Input: dimensioned drawing with shaded views. Units: mm. Origin: part minimum x, y, z. A direction names the side the tool comes from. Round coordinates to 2 decimals unless told otherwise and drop trailing zeros. Loops run counter-clockwise (first coordinate to the right, second up) from the corner with the lowest first, then second, coordinate; pieces in that order, holes last. Notation, with made-up numbers: (88, -23.75) - (146, -23.75) arc R23 cw to (146, 5.25) - close; hole circle Ø8 at (62.25, 53). An arc over 180 degrees is marked (long way). One line per question, with ' | ' between items. Start each with the question number.
Item 1: Section B-B, the plane x = 72.5. Return loops of the section in (y, z) (3 decimals), plus the area to 3 significant figures.
Item 2: Material intervals for line 1 along X through (y, z) = (7.5, 20); line 2 along X through (y, z) = (19, 20); line 3 along Z through (x, y) = (78.5, 20.5), sorted ascending.
Item 3: Draft query along Z for the marked faces 1, 2, 3 and 4. Return one class per face: pulls with the +Z half, pulls with the -Z half, needs draft (parallel to the pull), parting line crosses it, or undercut.
Item 4: Section C-C, the plane z = 5.5. Return loops of the section in (x, y) (3 decimals).
Item 5: First-contact query: pin 1 (14.5 mm diameter, centred on x = 80, z = 20, fed in from +Y); pin 2 (3 mm diameter, centred on y = 9.5, z = 23.5, fed in from -X); pin 3 (5 mm diameter, centred on y = 17, z = 29.5, fed in from +X) (3 decimals). Flat tips, straight axial feed; report the tip coordinate or a pass-through.
Item 6: Set-up query: the marked faces 5 and 6. Return all of +Z, -Z, +X, -X, +Y, -Y with unobstructed straight access to the full face (end or side cutting, diameter ignored); none if empty.
Item 7: Section A-A, the plane y = 13.75. Give the number of separate pieces and of enclosed holes in the cut face, plus the area to 3 significant figures.
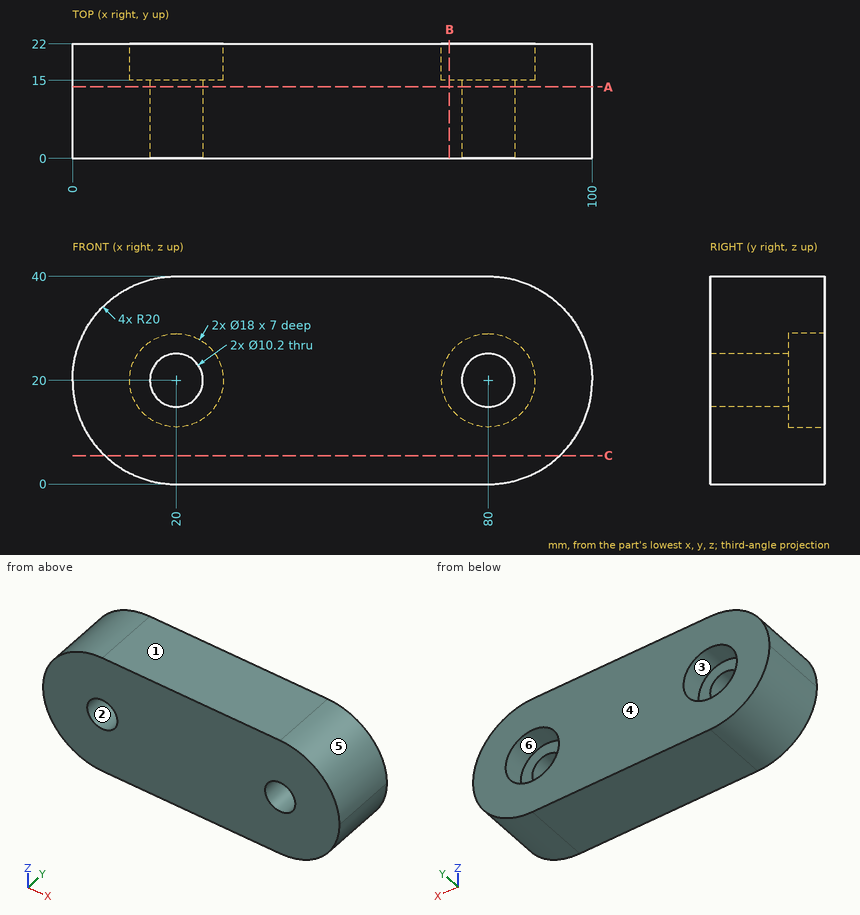
Return value:
1) outline: (0, 0) - (22, 0) - (22, 15.025) - (15, 15.025) - (15, 24.975) - (22, 24.975) - (22, 40) - (0, 40) - close | area: 810 mm2
2) line 1: 0 to 14.9, 25.1 to 74.9, 85.1 to 100 | line 2: 0 to 11, 29 to 71, 89 to 100 | line 3: 0 to 11.13, 28.87 to 40
3) face 1: pulls with the +Z half | face 2: undercut | face 3: undercut | face 4: needs draft
4) outline: (6.225, 0) - (93.775, 0) - (93.775, 22) - (6.225, 22) - close
5) pin 1: y = 15 | pin 2: x = 0.1 | pin 3: x = 98.735
6) face 5: +Z, +X, +Y, -Y | face 6: +Y
7) separate pieces: 1 | enclosed holes: 2 | area: 3,490 mm2
